Can you work these out from the model? Positions are in its coordinate system, mm. Give positions to 0.01 mm unless a question says otherwise; leave off trailing zeros. Loops run counter-clockwise (first coordinate to the right, second up) from the corner with the lowest first, then second, coordinate; pieces in that order, holes last. Notation, with made-up numbers: (-4, 1) -> (35, 1) arc R22 cw to (35, 40) -> close; hole circle Ø5 at (21.25, 62). An arc over 180 degrees is marked (long way). Return JSON: item names as keys, results as strings. Group by question number.
Q1. I need wall thicknesses on line 1 along X through (y, z) = (193.5, 0.4); line 2 along Y through (x, z) = (8, 0.5); line 3 along Y through (x, z) = (10.5, 0.15). Which ranges of each line are inside material? Lowest first, please. Write a range as [from, to].
Q2. Suppose I cut it at B-B, the plane y = 193.5. Please give me the cut outline in (x, z), and give its area (3 significant figures).
Q3. Suppose I cut it at A-A, the plane z = 0.25. Count the separate pieces of the cut face and the enclosed holes in it, and give its area (3 significant figures).
Q4. Suppose I cut it at C-C, the plane y = 5.4. Please give me the cut outline in (x, z).
Q5. Suppose I cut it at D-D, the plane y = 64.5. Please give me the cut outline in (x, z).
Q6. Will this pin go through, and if not, where does the flat tip stop? pin 1 (3.5 mm diameter, centred on x = 31.25, y = 14.4, fed in from +Z).
```python
from build123d import *

# Parameters (mm, degrees)
BOSS_EXTRUDE1_DEPTH = 0.6096
SKETCH3_R           = 1.7
SKETCH3_R_2         = 2.25
CUT_EXTRUDE1_DEPTH  = 204.304258716
SKETCH4_W           = 18.25
SKETCH4_H           = 57.225
BOSS_EXTRUDE2_DEPTH = 0.6096


with BuildPart() as part:
    # Sketch2 → Boss-Extrude1 (new body)
    with BuildSketch(Plane.XY):
        with BuildLine():
            Line((34.883504, 3.686554855), (36.164103759, 7.513864099))
            ThreePointArc((36.164103759, 7.513864099), (36.415476383, 8.531517689), (36.5, 9.576344365))
            Line((36.5, 9.576344365), (36.5, 198))
            ThreePointArc((36.5, 198), (35.914213562, 199.414213562), (34.5, 200))
            Line((34.5, 200), (2, 200))
            ThreePointArc((2, 200), (0.585786438, 199.414213562), (0, 198))
            Line((0, 198), (0, 9.576344365))
            ThreePointArc((0, 9.576344365), (0.084523617, 8.531517689), (0.335896241, 7.513864099))
            Line((0.335896241, 7.513864099), (1.616496, 3.686554855))
            ThreePointArc((1.616496, 3.686554855), (3.582495544, 1.017500497), (6.737443738, 0))
            Line((6.737443738, 0), (29.762556262, 0))
            ThreePointArc((29.762556262, 0), (32.917504456, 1.017500497), (34.883504, 3.686554855))
        make_face()
    extrude(amount=BOSS_EXTRUDE1_DEPTH)

    # Sketch3 → Cut-Extrude1 (cut, through all)
    with BuildSketch(Plane.XY.offset(0.6096)):
        with Locations((8.25, 5.4)):
            Circle(SKETCH3_R)
        with Locations((5.25, 14.4)):
            Circle(SKETCH3_R_2)
        with Locations((10.75, 193.5)):
            Circle(SKETCH3_R_2)
        with Locations(Location((28.25, 5.4, 0), (0, 0, 180))):
            Circle(SKETCH3_R)
        with Locations(Location((31.25, 14.4, 0), (0, 0, 180))):
            Circle(SKETCH3_R_2)
        with Locations(Location((25.75, 193.5, 0), (0, 0, 180))):
            Circle(SKETCH3_R_2)
    extrude(amount=-CUT_EXTRUDE1_DEPTH, mode=Mode.SUBTRACT)

    # Sketch4 → Boss-Extrude2 (add)
    with BuildSketch(Plane.XY.offset(0.6096)):
        with Locations((9.125, 100.6125)):
            Rectangle(SKETCH4_W, SKETCH4_H)
        with BuildLine():
            ThreePointArc((0, 129.225), (-6.75, 100.6125), (0, 72))
            Line((0, 72), (0, 129.225))
        make_face()
        with Locations((27.375, 100.6125)):
            Rectangle(SKETCH4_W, SKETCH4_H)
        with BuildLine():
            Line((36.5, 129.225), (36.5, 72))
            ThreePointArc((36.5, 72), (43.25, 100.6125), (36.5, 129.225))
        make_face()
    extrude(amount=-BOSS_EXTRUDE2_DEPTH)


solid = part.part
```
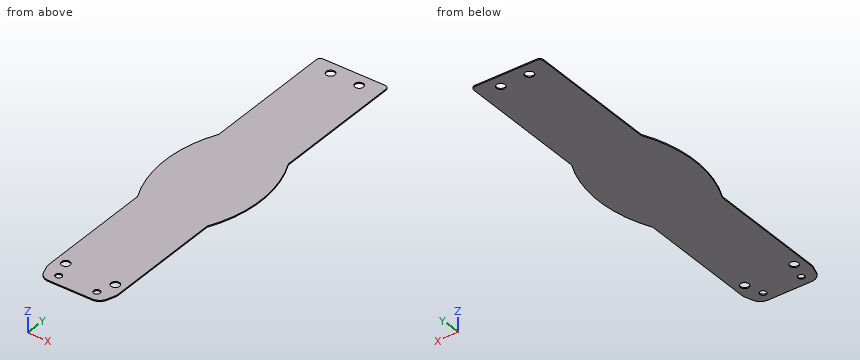
Ans:
{
 "1": {"line 1": "x = [0, 8.5], [13, 23.5], [28, 36.5]", "line 2": "y = [0, 3.72], [7.08, 200]", "line 3": "y = [0, 191.26], [195.74, 200]"},
 "2": {"outline": "(0, 0) -> (8.5, 0) -> (8.5, 0.61) -> (0, 0.61) -> close; (13, 0) -> (23.5, 0) -> (23.5, 0.61) -> (13, 0.61) -> close; (28, 0) -> (36.5, 0) -> (36.5, 0.61) -> (28, 0.61) -> close", "area": "16.8 mm^2"},
 "3": {"separate pieces": "1", "enclosed holes": "6", "area": "7,710 mm^2"},
 "4": {"outline": "(1.04, 0) -> (6.55, 0) -> (6.55, 0.61) -> (1.04, 0.61) -> close; (9.95, 0) -> (26.55, 0) -> (26.55, 0.61) -> (9.95, 0.61) -> close; (29.95, 0) -> (35.46, 0) -> (35.46, 0.61) -> (29.95, 0.61) -> close"},
 "5": {"outline": "(0, 0) -> (36.5, 0) -> (36.5, 0.61) -> (0, 0.61) -> close"},
 "6": {"pin 1": "passes through"}
}
